from build123d import *

# Parameters (mm, degrees)
SKETCH_W     = 80
SKETCH_H     = 60
PAD_DEPTH    = 10
POCKET_DEPTH = 7
FILLET001_R  = 10
SKETCH003_W  = 19.974239
SKETCH003_H  = 0.973365
PAD001_DEPTH = 2


with BuildPart() as part:
    # Sketch → Pad (new body)
    with BuildSketch(Plane.XY):
        Rectangle(SKETCH_W, SKETCH_H)
    extrude(amount=PAD_DEPTH)

    # Sketch002 (on Face6 of Pad) → Pocket (cut)
    with BuildSketch(Plane.XY.offset(10)):
        Polygon((-28, 27), (28, 27), (37, 20.000019), (37, -20.000019), (28, -27), (-28, -27), (-37, -20.000019), (-37, 20.000019), align=None)
    extrude(amount=-POCKET_DEPTH, mode=Mode.SUBTRACT)

    # Fillet001
    fillet001_edges = [part.edges().sort_by_distance(p)[0] for p in [
        (-40, 30, 5),
        (40, 30, 5),
        (40, -30, 5),
        (-40, -30, 5),
    ]]
    fillet(fillet001_edges, radius=FILLET001_R)

    # Sketch003 (on Face6 of Fillet001) → Pad001 (join)
    with BuildSketch(Plane(origin=(-40, 0, 0), x_dir=(0, -1, 0), z_dir=(-1, 0, 0))):
        with Locations((-0.012881, 9.513317)):
            Rectangle(SKETCH003_W, SKETCH003_H)
    pad001 = extrude(amount=PAD001_DEPTH)

    # Mirrored: Pad001 across YZ
    add(pad001.mirror(Plane.YZ))


solid = part.part
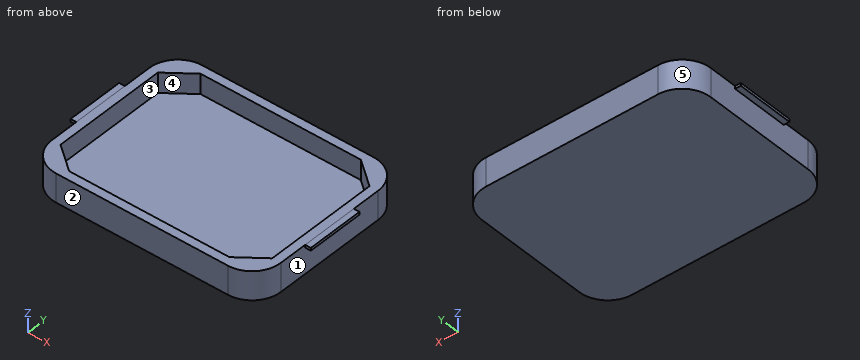
Verification items for the finished model (mm, model axes). Face numbers are marked on the shaded views. A direction names the side the tool comes from. Coordinates: 2 decimals unless noted, no trailing zeros. Loops run counter-clockwise (first coordinate to the right, second up) from the corner with the lowest first, then second, coordinate; pieces in that order, holes last. Notation, with made-up numbers: M -16.5,29.25 L 15.5,29.25 A20 ccw 15.5,37.25 Z; hole C -40,68.5 d4. An arc over 180 degrees is marked long. One line per item, written item: value.
1. Section check A-A on z = 6.5. Record the cut outline in (x, y), plus the area to 3 significant figures.
Answers follow:
outline: M -40,-20 A10 ccw -30,-30 L 30,-30 A10 ccw 40,-20 L 40,20 A10 ccw 30,30 L -30,30 A10 ccw -40,20 Z; hole M -37,-20 L -28,-27 L 28,-27 L 37,-20 L 37,20 L 28,27 L -28,27 L -37,20 Z
area: 844 mm^2
2. Gauge pin test, flat ends, axial feed: P1, Ø0.6, axis at x = 40.5, y = 2, coming from the -Z side; P2, Ø1.1, axis at x = -41.5, z = 10, coming from the +Y side; P3, Ø3, axis at y = -6.5, z = 4, coming from the -X side. Record the tip position at first contact, or that the pin passes through.
Answers follow:
P1: z = 9.03
P2: y = 10
P3: x = -40
3. Material ranges on line 1 along Y through (x, z) = (-16.5, 9.5); line 2 along X through (y, z) = (6.5, 9.5); line 3 along X through (y, z) = (9, 4), recorded low to high. Write a range as from..to.
Answers follow:
line 1: -30..-27, 27..30
line 2: -42..-37, 37..42
line 3: -40..-37, 37..40
4. Mould release check, pull along Y, two halves, no side actions. Record for the marked faces 1, 2 and 3: pulls with the +Y half, pulls with the -Y half, needs draft (parallel to the pull), parting line crosses it, or undercut.
Answers follow:
face 1: needs draft
face 2: pulls with the -Y half
face 3: undercut
5. Section check B-B on z = 1. Record the cut outline in (x, y), plus the area to 3 significant figures.
Answers follow:
outline: M -40,-20 A10 ccw -30,-30 L 30,-30 A10 ccw 40,-20 L 40,20 A10 ccw 30,30 L -30,30 A10 ccw -40,20 Z
area: 4,710 mm^2
6. Set-up check for the marked faces 4 and 5: record each of +Z, -Z, +X, -X, +Y, -Y from which the full face is reachable in a straight line by a thin tool's end or side.
Answers follow:
face 4: +Z
face 5: +Z, -Z, -X, +Y
7. Section check C-C on x = -17.5. Record the cut outline in (y, z), plus the area to 3 significant figures.
Answers follow:
outline: M -30,0 L 30,0 L 30,10 L 27,10 L 27,3 L -27,3 L -27,10 L -30,10 Z
area: 222 mm^2
8. Section check D-D on y = 5.5. Record the cut outline in (x, z), plus the area to 3 significant figures.
Answers follow:
outline: M -42,9.03 L -40,9.03 L -40,0 L 40,0 L 40,9.03 L 42,9.03 L 42,10 L 37,10 L 37,3 L -37,3 L -37,10 L -42,10 Z
area: 286 mm^2
